Here's how the part is built. I have some questions about the finished solid (model axes, mm). A direction names the side the tool comes from. Round coordinates to 2 decimals unless told otherwise and drop trailing zeros. Loops run counter-clockwise (first coordinate to the right, second up) from the corner with the lowest first, then second, coordinate; pieces in that order, holes last. Notation, with made-up numbers: M -7,19.5 L 27,19.5 A17 ccw 27,47.5 Z; hole C 22.5,14.5 d3. An arc over 180 degrees is marked long. Answer as a JSON object with one key per item and string values.
from build123d import *

# Parameters (mm, degrees)
F0_R     = 19.304886182
F1_DEPTH = 31.496
F2_R     = 6.7453126933
F3_T     = -2.54


# Not quite as in the source:
# - a shell that OpenCascade refuses in one call is made with other operations: the cavity is built on its own and cut out


with BuildPart() as f1:
    # F0 (on Front) → F1 (new body)
    with BuildSketch(Plane.XZ):
        with Locations((-28.4389294684, 24.6289279312)):
            Circle(F0_R)
    extrude(amount=F1_DEPTH)

    # F2
    f2_edges = [f1.edges().sort_by_distance(p)[0] for p in [
        (-47.743816, -31.496, 24.628928),
    ]]
    fillet(f2_edges, radius=F2_R)

    # F3: a shell. OpenCascade refuses it in one call, so the cavity is built on its own and cut out:
    # the body offset inwards by the wall thickness, plus a prism from it out through each open face.
    f3_core = offset(f1.part, amount=F3_T, mode=Mode.PRIVATE)
    f3_exits = [f3_core.faces().sort_by_distance(p)[0] for p in [
        (-28.438929, -28.956, 24.628928),
    ]]
    add(f3_core, mode=Mode.SUBTRACT)
    extrude(f3_exits, amount=-F3_T, mode=Mode.SUBTRACT)


solid = f1.part
Item 1: I'm going to push flat-ended pins straight in: pin 1 Ø6 at (x, y) = (-29.5, -12.5) entering from +Z; pin 2 Ø3 at (y, z) = (-24.5, 17) entering from -X; pin 3 Ø1.5 at (x, y) = (-17, -20.5) entering from +Z. Where does each tip first touch, or does it pass through?
Resolved:
{"pin 1": "z = 43.93", "pin 2": "x = -46.75", "pin 3": "z = 40.7"}
Item 2: I want a section at A-A, the plane y = -20. Please give me the cut outline in (x, z), then the cut area to 3 significant figures.
Resolved:
{"outline": "C -28.44,24.63 d38.61; hole C -28.44,24.63 d33.53", "area": "288 mm²"}
Item 3: On a 3-axis mill with a long thin cutter (end or side, diameter ignored), from which of +Z, -Z, +X, -X, +Y, -Y can I reach the whole of each face in a straight line? I mean faces 1 (the face through (-21.69, -30.21, 35.22)), 2 (the face through (-29, -2.54, 25)). Say none if no direction works.
Resolved:
{"face 1": "-Y", "face 2": "none"}
Item 4: If we mould it in two halves opening along X, with no side actions, what happens to faces 3 (the face through (-29, 0, 25)), 4 (the face through (-12.448, -13.49, 29.665)), 5 (the face through (-19.531, -12.202, 7.502))? For each: pulls with the +X half, pulls with the -X half, needs draft (parallel to the pull), parting line crosses it, or undercut.
Resolved:
{"face 3": "needs draft", "face 4": "undercut", "face 5": "parting line crosses it"}
Item 5: Please list where these lines run through material, in increasing order: probe 1 along Z at (x, y) = (-28.5, -14); probe 2 along X at (y, z) = (-23.5, 25); probe 3 along Y at (x, z) = (-33.5, 29). Write a range as from..to.
Resolved:
{"probe 1": "5.32..7.86, 41.39..43.93", "probe 2": "-47.74..-45.2, -11.68..-9.14", "probe 3": "-2.54..0"}
